Geometry check sheet. Reference: drawing and pictorial views, mm from the part's lowest x, y, z. A direction names the side the tool comes from. Round coordinates to 2 decimals unless told otherwise and drop trailing zeros. Write each loop counter-clockwise with the first axis right and the second up, starting at its lowest first coordinate (ties: lowest second). Pieces come first, ordered by that corner, then holes. Notation, with made-up numbers: (86.5, 81.25) -> (118.5, 81.25) arc R20 ccw to (118.5, 94.25) -> close; hole circle Ø11 at (1, -34). An arc over 180 degrees is marked (long way). Answer as a JSON object with one key per item and string values. Group by question number.
(1) Sectioned sample at D-D on x = 15. Record the cut outline in (y, z), and give its area (3 significant figures).
(2) Sectioned sample at B-B on y = 10. Record the cut outline in (x, z), and give its area (3 significant figures).
(3) Set-up check for the marked faces 1, 2 and 3: record each of +Z, -Z, +X, -X, +Y, -Y from which the full face is reachable in a straight line by a thin tool's end or side.
(4) Scan lines: L1, parallel to Z at x = 1.55, y = 10; L2, parallel to X at y = 18, z = 9.5; L3, parallel to X at y = 52.5, z = 15.25 (1 decimal). Record each from-to range of solid material in increasing order. Write a range as from..to.
(5) Gauge pin test, flat ends, axial feed: pin 1 Ø11 at (y, z) = (10, 15.02) entering from +X; pin 2 Ø8 at (x, y) = (20.5, 60) entering from -Z; pin 3 Ø15 at (y, z) = (32.5, 13.5) entering from -X; pin 4 Ø7 at (x, z) = (11.5, 20) entering from -Y. Record the tip position at first contact, or that the pin passes through.
(6) Sectioned sample at A-A on y = 22.5. Record the cut outline in (x, z).
(7) Draft check along X on the marked faces 4, 5 and 6. Enter one of: released by +X, released by -X, zero draft, split by the parting line, or undercut.
(8) Sectioned sample at C-C on z = 23. Record the cut outline in (x, y), and give its area (3 significant figures).
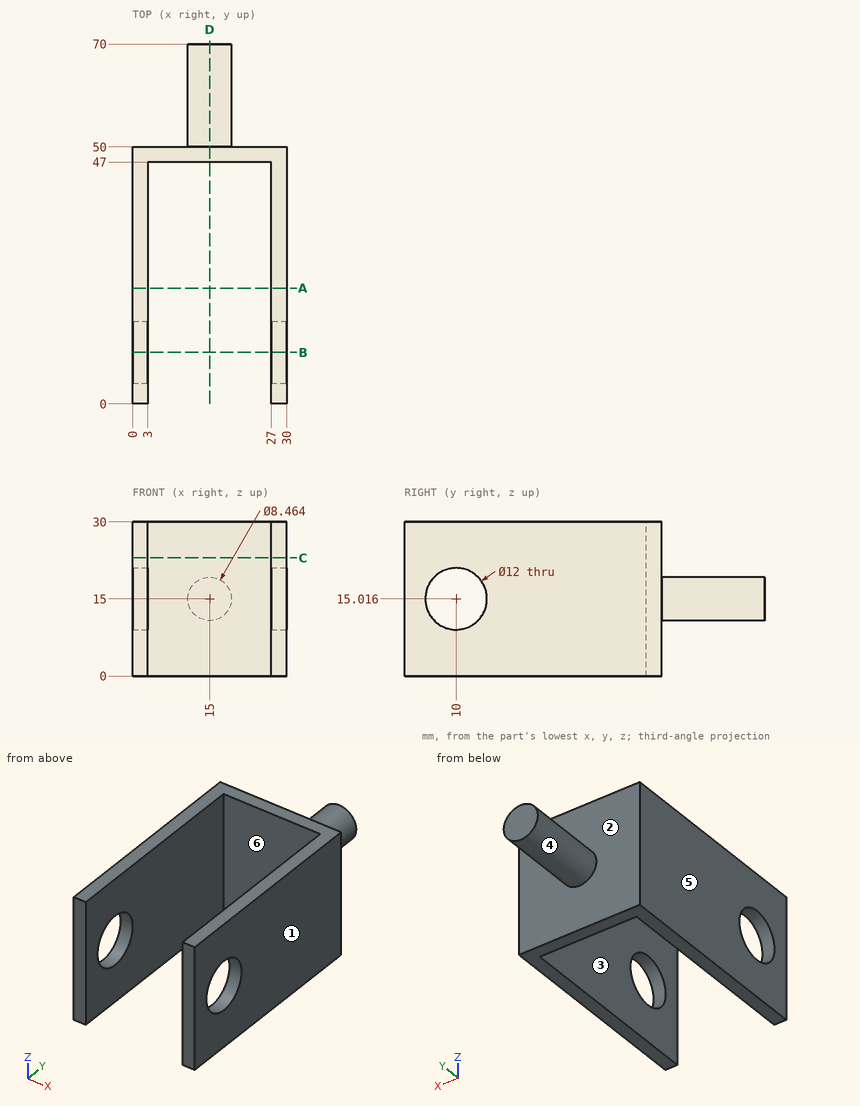
Computed values:
{
 "1": {"outline": "(47, 0) -> (50, 0) -> (50, 10.77) -> (70, 10.77) -> (70, 19.23) -> (50, 19.23) -> (50, 30) -> (47, 30) -> close", "area": "259 mm2"},
 "2": {"outline": "(0, 0) -> (3, 0) -> (3, 9.02) -> (0, 9.02) -> close; (0, 21.02) -> (3, 21.02) -> (3, 30) -> (0, 30) -> close; (27, 0) -> (30, 0) -> (30, 9.02) -> (27, 9.02) -> close; (27, 21.02) -> (30, 21.02) -> (30, 30) -> (27, 30) -> close", "area": "108 mm2"},
 "3": {"face 1": "+Z, -Z, +X, +Y, -Y", "face 2": "+Y", "face 3": "+Z, -Z, -Y"},
 "4": {"L1": "0..9.02, 21.02..30", "L2": "0..3, 27..30", "L3": "10.8..19.2"},
 "5": {"pin 1": "through", "pin 2": "z = 11.04", "pin 3": "x = 0", "pin 4": "y = 47"},
 "6": {"outline": "(0, 0) -> (3, 0) -> (3, 30) -> (0, 30) -> close; (27, 0) -> (30, 0) -> (30, 30) -> (27, 30) -> close"},
 "7": {"face 4": "split by the parting line", "face 5": "released by -X", "face 6": "undercut"},
 "8": {"outline": "(0, 0) -> (3, 0) -> (3, 47) -> (27, 47) -> (27, 0) -> (30, 0) -> (30, 50) -> (0, 50) -> close", "area": "372 mm2"}
}
